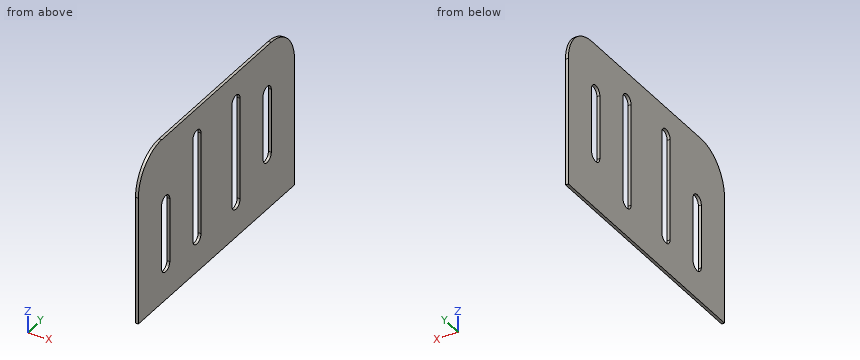
from build123d import *

# Parameters (mm, degrees)
F1_DEPTH = 4.5


with BuildPart() as f1:
    # F0 (on Right) → F1 (new body)
    with BuildSketch(Plane.YZ):
        with BuildLine():
            Line((-100, -710), (300, -710))
            Line((300, -710), (300, -510))
            ThreePointArc((300, -510), (282.426407, -467.573593), (240, -450))
            Line((240, -450), (-40, -450))
            ThreePointArc((-40, -450), (-82.426407, -467.573593), (-100, -510))
            Line((-100, -510), (-100, -710))
        make_face()
        with BuildLine():
            ThreePointArc((-19.5, -655), (-30, -665.5), (-40.5, -655))
            Line((-40.5, -655), (-40.5, -555))
            ThreePointArc((-40.5, -555), (-30, -544.5), (-19.5, -555))
            Line((-19.5, -555), (-19.5, -655))
        make_face(mode=Mode.SUBTRACT)
        with BuildLine():
            Line((39.5, -655), (39.5, -495))
            ThreePointArc((39.5, -495), (50, -484.5), (60.5, -495))
            Line((60.5, -495), (60.5, -655))
            ThreePointArc((60.5, -655), (50, -665.5), (39.5, -655))
        make_face(mode=Mode.SUBTRACT)
        with BuildLine():
            Line((139.5, -655), (139.5, -495))
            ThreePointArc((139.5, -495), (150, -484.5), (160.5, -495))
            Line((160.5, -495), (160.5, -655))
            ThreePointArc((160.5, -655), (150, -665.5), (139.5, -655))
        make_face(mode=Mode.SUBTRACT)
        with BuildLine():
            ThreePointArc((240.5, -625), (230, -635.5), (219.5, -625))
            Line((219.5, -625), (219.5, -525))
            ThreePointArc((219.5, -525), (230, -514.5), (240.5, -525))
            Line((240.5, -525), (240.5, -625))
        make_face(mode=Mode.SUBTRACT)
    extrude(amount=-F1_DEPTH)


solid = f1.part
Work out the finished part from the listing and answer in its coordinate system (mm). Round coordinates to 2 decimals unless told otherwise and drop trailing zeros. Write each loop counter-clockwise with the first axis right and the second up, starting at its lowest first coordinate (ties: lowest second). Pieces come first, ordered by that corner, then holes. Notation, with made-up numbers: (23.25, -11) -> (69.25, -11) arc R27 ccw to (69.25, 10) -> close; hole circle Ø8 at (16, 66.5). An arc over 180 degrees is marked (long way). Answer as CSV lines item,"result". Start each with the question number.
(1) The part is cut by section B-B, the plane y = 50. Give the vertices of the cut face in (x, z).
(2) The part is cut by section C-C, the plane z = -590. Give the vertices of the cut face in (x, y), then the cut area to 3 significant figures.
(3) Find the intervals of material crossed by probe 1 along Y at (x, z) = (-2.35, -527); probe 2 along Y at (x, z) = (-1.2, -602.5); probe 3 along Y at (x, z) = (-0.5, -640.5), in increasing order.
(4) The part is cut by section A-A, the plane z = -646.5. Give the vertices of the cut face in (x, y), then the cut area to 3 significant figures.
(5) The part is cut by section D-D, the plane x = -1.95. Give the vertices of the cut face in (y, z).
Output values:
1,outline,"(-4.5, -710) -> (0, -710) -> (0, -665.5) -> (-4.5, -665.5) -> close; (-4.5, -484.5) -> (0, -484.5) -> (0, -450) -> (-4.5, -450) -> close"
2,outline,"(-4.5, -100) -> (0, -100) -> (0, -40.5) -> (-4.5, -40.5) -> close; (-4.5, -19.5) -> (0, -19.5) -> (0, 39.5) -> (-4.5, 39.5) -> close; (-4.5, 60.5) -> (0, 60.5) -> (0, 139.5) -> (-4.5, 139.5) -> close; (-4.5, 160.5) -> (0, 160.5) -> (0, 219.5) -> (-4.5, 219.5) -> close; (-4.5, 240.5) -> (0, 240.5) -> (0, 300) -> (-4.5, 300) -> close"
2,area,"1,420 mm²"
3,probe 1,"y = -100 to 39.5, 60.5 to 139.5, 160.5 to 219.5, 240.5 to 300"
3,probe 2,"y = -100 to -40.5, -19.5 to 39.5, 60.5 to 139.5, 160.5 to 219.5, 240.5 to 300"
3,probe 3,"y = -100 to -40.5, -19.5 to 39.5, 60.5 to 139.5, 160.5 to 300"
4,outline,"(-4.5, -100) -> (0, -100) -> (0, -40.5) -> (-4.5, -40.5) -> close; (-4.5, -19.5) -> (0, -19.5) -> (0, 39.5) -> (-4.5, 39.5) -> close; (-4.5, 60.5) -> (0, 60.5) -> (0, 139.5) -> (-4.5, 139.5) -> close; (-4.5, 160.5) -> (0, 160.5) -> (0, 300) -> (-4.5, 300) -> close"
4,area,"1,520 mm²"
5,outline,"(-100, -710) -> (300, -710) -> (300, -510) arc R60 ccw to (240, -450) -> (-40, -450) arc R60 ccw to (-100, -510) -> close; hole (-40.5, -655) arc R10.5 ccw to (-19.5, -655) -> (-19.5, -555) arc R10.5 ccw to (-40.5, -555) -> close; hole (39.5, -655) arc R10.5 ccw to (60.5, -655) -> (60.5, -495) arc R10.5 ccw to (39.5, -495) -> close; hole (139.5, -655) arc R10.5 ccw to (160.5, -655) -> (160.5, -495) arc R10.5 ccw to (139.5, -495) -> close; hole (219.5, -625) arc R10.5 ccw to (240.5, -625) -> (240.5, -525) arc R10.5 ccw to (219.5, -525) -> close"
